```python
from build123d import *

# Parameters (mm, degrees)
F0_W     = 4.4
F0_H     = 9
F0_R     = 1.25
F1_DEPTH = 3
F2_W     = 44.8
F2_H     = 7.4952778638
F2_R     = 1.778
F3_DEPTH = 3
F4_R     = 2
F5_R     = 2


with BuildPart() as f1:
    # F0 (on Front) → F1 (new body)
    with BuildSketch(Plane.XZ):
        with Locations((2.2, 4.5)):
            Rectangle(F0_W, F0_H)
        with Locations((2.2, 6)):
            Circle(F0_R, mode=Mode.SUBTRACT)
    extrude(amount=F1_DEPTH)



with BuildPart() as f1b:
    # F0 (on Front) → F1, piece 2 (new body)
    with BuildSketch(Plane.XZ):
        with Locations((28.6, 4.5)):
            Rectangle(F0_W, F0_H)
        with Locations((28.6, 6)):
            Circle(F0_R, mode=Mode.SUBTRACT)
    extrude(amount=F1_DEPTH)


with BuildPart() as f1_1:
    add(f1.part)

    add(f1b.part)  # F3 merges F1b
    # F2 (on Top) → F3 (join)
    with BuildSketch(Plane.XY):
        with Locations((15.4, 0.7476389319)):
            Rectangle(F2_W, F2_H)
        with Locations((-3.5, 1.5)):
            Circle(F2_R, mode=Mode.SUBTRACT)
        with Locations((34.3, 1.5)):
            Circle(F2_R, mode=Mode.SUBTRACT)
    extrude(amount=-F3_DEPTH)

    # F4
    f4_edges = [f1_1.edges().sort_by_distance(p)[0] for p in [
        (0, -1.5, 0),
        (4.4, -1.5, 0),
        (26.4, -1.5, 0),
        (30.8, -1.5, 0),
    ]]
    fillet(f4_edges, radius=F4_R)

    # F5
    f5_edges = [f1_1.edges().sort_by_distance(p)[0] for p in [
        (-7, -3, -1.5),
        (-7, 4.495278, -1.5),
        (37.8, -3, -1.5),
        (37.8, 4.495278, -1.5),
    ]]
    fillet(f5_edges, radius=F5_R)


solid = f1_1.part
```
Design review of the part built by this model. Coordinates are the model's own, in mm. A direction names the side the tool comes from. Give positions to 0.01 mm unless a question says otherwise; leave off trailing zeros. Loops run counter-clockwise (first coordinate to the right, second up) from the corner with the lowest first, then second, coordinate; pieces in that order, holes last. Notation, with made-up numbers: M 74,64.25 L 93,64.25 A25 cw 93,100.25 Z; hole C 57.5,-25 d6. An arc over 180 degrees is marked long. Return JSON: item names as keys, results as strings. Group by question number.
Item 1: Insertion check: pin 1 Ø0.9 at (y, z) = (-2, 7) entering from +X; pin 2 Ø3.5 at (y, z) = (-1, 4.5) entering from -X; pin 3 Ø6.5 at (x, z) = (28, 5.5) entering from +Y. Each pin has a flat end and moves straight along its axis. Give the tip position at first contact, or say it passes through.
Item 2: Tool access review of faces 1 (the flat face through (30.8, -1, 5)), 2 (the flat face through (4.4, -1, 5)), 3 (the flat face through (15, 2, 0)): name each direction out of +Z, -Z, +X, -X, +Y, -Y from which nothing blocks a thin tool from reaching the whole face with its end or side.
Item 3: We need section C-C (x = 28.6). Give the boundary of the cut face in (y, z), and give its area (3 significant figures).
Item 4: For probe 1 along X at (y, z) = (-1.75, 4); probe 2 along Y at (x, z) = (34.3, -1.1); probe 3 along Z at (x, y) = (2.2, -1.9), list the stretches that pass through material, from the lowest coordinate up.
Item 5: We need section D-D (y = -2). Give the boundary of the cut face in (x, z), and give its area (3 significant figures).
Item 6: We need section A-A (z = 3.75). Give the boundary of the cut face in (x, y).
Item 7: We need section B-B (y = 1.5). Give the boundary of the cut face in (x, z), and give its area (3 significant figures).
Item 8: Mouldability with a two-part tool opening along X and no side actions: class faces 4 (the cylindrical face through (32.524, 1.578, -1.479)), 5 (the cylindrical face through (31.4, -1.52, 0.57)), 6 (the flat face through (0, -1, 5)), 7 (the flat face through (15, 4.495, -1)) as released by +X, released by -X, zero draft, split by the parting line, or undercut.
Output:
{
 "1": {"pin 1": "stops at x = 30.8", "pin 2": "stops at x = 0", "pin 3": "stops at y = 0"},
 "2": {"face 1": "+Z, +X, +Y, -Y", "face 2": "+Z, +Y, -Y", "face 3": "+Z, +Y"},
 "3": {"outline": "M -3,-3 L 4.5,-3 L 4.5,0 L 0,0 L 0,4.75 L -3,4.75 Z; M -3,7.25 L 0,7.25 L 0,9 L -3,9 Z", "area": "42.0 mm^2"},
 "4": {"probe 1": "x = 0 to 4.4, 26.4 to 30.8", "probe 2": "y = -3 to -0.28, 3.28 to 4.5", "probe 3": "z = -3 to 4.75, 7.25 to 9"},
 "5": {"outline": "M -6.73,-3 L 37.53,-3 L 37.53,0 L 32.8,0 A2 cw 30.8,2 L 30.8,9 L 26.4,9 L 26.4,2 A2 cw 24.4,0 L 6.4,0 A2 cw 4.4,2 L 4.4,9 L 0,9 L 0,2 A2 cw -2,0 L -6.73,0 Z; hole C 2.2,6 d2.5; hole C 28.6,6 d2.5", "area": "206 mm^2"},
 "6": {"outline": "M 0,-3 L 4.4,-3 L 4.4,0 L 0,0 Z; M 26.4,-3 L 30.8,-3 L 30.8,0 L 26.4,0 Z"},
 "7": {"outline": "M -7,-3 L -5.28,-3 L -5.28,0 L -7,0 Z; M -1.72,-3 L 32.52,-3 L 32.52,0 L -1.72,0 Z; M 36.08,-3 L 37.8,-3 L 37.8,0 L 36.08,0 Z", "area": "113 mm^2"},
 "8": {"face 4": "undercut", "face 5": "released by +X", "face 6": "released by -X", "face 7": "zero draft"}
}
